```python
from build123d import *

# Parameters (mm, degrees)
SKETCH1_W           = 75.565
SKETCH1_H           = 22.86
BOSS_EXTRUDE1_DEPTH = 5.08
SKETCH2_W           = 35.56
SKETCH2_H           = 17.78
CUT_EXTRUDE1_DEPTH  = 2.54
SKETCH3_W           = 34.925
SKETCH3_H           = 12.7
CUT_EXTRUDE2_DEPTH  = 40.799103083


with BuildPart() as part:
    # Sketch1 → Boss-Extrude1 (new body)
    with BuildSketch(Plane.XY):
        Rectangle(SKETCH1_W, SKETCH1_H)
    extrude(amount=BOSS_EXTRUDE1_DEPTH)

    # Sketch2 → Cut-Extrude1 (cut)
    with BuildSketch(Plane.XY.offset(5.08)):
        with Locations((-17.4625, 0)):
            Rectangle(SKETCH2_W, SKETCH2_H)
    extrude(amount=-CUT_EXTRUDE1_DEPTH, mode=Mode.SUBTRACT)

    # Sketch3 → Cut-Extrude2 (cut, through all)
    with BuildSketch(Plane.XY.offset(5.08)):
        with Locations((17.78, 0)):
            Rectangle(SKETCH3_W, SKETCH3_H)
    extrude(amount=-CUT_EXTRUDE2_DEPTH, mode=Mode.SUBTRACT)


solid = part.part
```
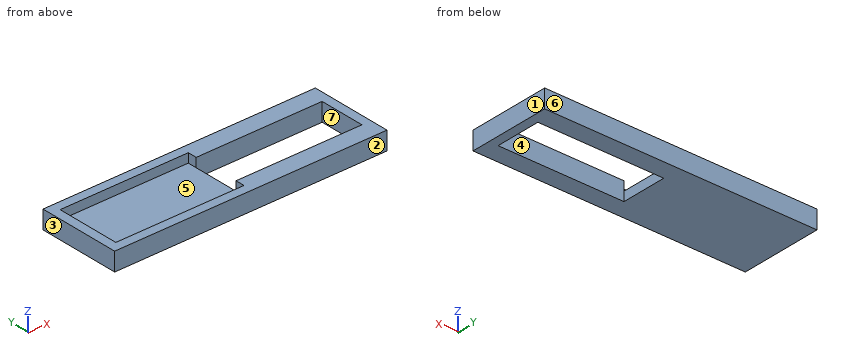
Model file for the job. Use its own axes, mm. Face numbers are marked on the shaded views. A direction names the side the tool comes from. Round coordinates to 2 decimals unless told otherwise and drop trailing zeros. Write each loop counter-clockwise with the first axis right and the second up, starting at its lowest first coordinate (ties: lowest second). Pieces come first, ordered by that corner, then holes. Notation, with made-up numbers: (84, 89.25) - (114, 89.25) arc R27 ccw to (114, 120.25) - close; hole circle Ø6 at (54, -23.75). An arc over 180 degrees is marked (long way). One line per item, written item: value.
(1) 3-axis set-ups, long thin cutter, end or side, ignore diameter. For the marked faces 5, 6 and 7: which of +Z, -Z, +X, -X, +Y, -Y reach the whole face in a straight line?
Values follow:
face 5: +Z
face 6: +Z, -Z, +X, -X, +Y
face 7: +Z, -Z
(2) Two-plate mould, pull along X, no slides. Class the marked faces 1, 2, 3 and 4: pulls with the +X half, pulls with the -X half, needs draft (parallel to the pull), parting line crosses it, or undercut.
Values follow:
face 1: pulls with the +X half
face 2: needs draft
face 3: pulls with the -X half
face 4: undercut
(3) Drop a flat-ended pin along its axis: P1, Ø5, axis at x = -30, y = -0.5, coming from the +Z side. Give the stop position or say it passes through.
Values follow:
P1: stops at z = 2.54
(4) Cut at B-B, the plane y = 1. Give the cut face in (x, z).
Values follow:
outline: (-37.78, 0) - (0.32, 0) - (0.32, 2.54) - (-35.24, 2.54) - (-35.24, 5.08) - (-37.78, 5.08) - close; (35.24, 0) - (37.78, 0) - (37.78, 5.08) - (35.24, 5.08) - close
(5) Cut at A-A, the plane x = 19. Give the cut face in (y, z), plus the area to 3 significant figures.
Values follow:
outline: (-11.43, 0) - (-6.35, 0) - (-6.35, 5.08) - (-11.43, 5.08) - close; (6.35, 0) - (11.43, 0) - (11.43, 5.08) - (6.35, 5.08) - close
area: 51.6 mm²
(6) Wall check: probe 1 along X at (y, z) = (3, 0.95); probe 2 along Y at (x, z) = (-30, 3.8); probe 3 along Y at (x, z) = (20.5, 3.8). Give the ranges that are in metal, low to high.
Values follow:
probe 1: x = -37.78 to 0.32, 35.24 to 37.78
probe 2: y = -11.43 to -8.89, 8.89 to 11.43
probe 3: y = -11.43 to -6.35, 6.35 to 11.43
(7) Cut at D-D, the plane x = -26. Give the cut face in (y, z).
Values follow:
outline: (-11.43, 0) - (11.43, 0) - (11.43, 5.08) - (8.89, 5.08) - (8.89, 2.54) - (-8.89, 2.54) - (-8.89, 5.08) - (-11.43, 5.08) - close
(8) Cut at C-C, the plane z = 3.75. Give the cut face in (x, y).
Values follow:
outline: (-37.78, -11.43) - (37.78, -11.43) - (37.78, 11.43) - (-37.78, 11.43) - close; hole (-35.24, -8.89) - (0.32, -8.89) - (0.32, -6.35) - (35.24, -6.35) - (35.24, 6.35) - (0.32, 6.35) - (0.32, 8.89) - (-35.24, 8.89) - close
